Source: CAD feature listing. Evaluate the final solid. Frame: model axes, mm. Give positions to 0.01 mm unless a question says otherwise; leave off trailing zeros. Write each loop counter-clockwise with the first axis right and the second up, starting at its lowest first coordinate (ties: lowest second). Pieces come first, ordered by that corner, then holes. Notation, with made-up numbers: (4, 64.25) -> (33, 64.25) arc R5 ccw to (33, 72.25) -> close; hole circle Ø11 at (-15.75, 55.5). An arc over 180 degrees is marked (long way). Answer as a JSON object with one key per item and string values. Group by question number.
Item 1: Section query A-A on y = 0.75. Return the cut outline in (x, z), plus the area to 3 significant figures.
Item 2: Ray query, probe 1 along Z at (x, y) = (26, 2); probe 2 along Z at (x, y) = (-1, 2); probe 3 along X at (y, z) = (0.45, -1.5) (1 decimal). Return the intervals inside material, ascending. Write a range as from..to.
Item 3: First-contact query: pin 1 Ø2 at (x, y) = (23.5, 2) entering from +Z; pin 2 Ø2 at (x, y) = (6.5, 1) entering from +Z. Flat tips, straight axial feed; report the tip coordinate or a pass-through.
Item 4: Section query B-B on x = 4. Return the cut outline in (y, z).
Item 5: Section query C-C on z = -35. Return the cut outline in (x, y), plus the area to 3 significant figures.
Item 6: Section query D-D on x = 36. Return the cut outline in (y, z), plus the area to 3 significant figures.
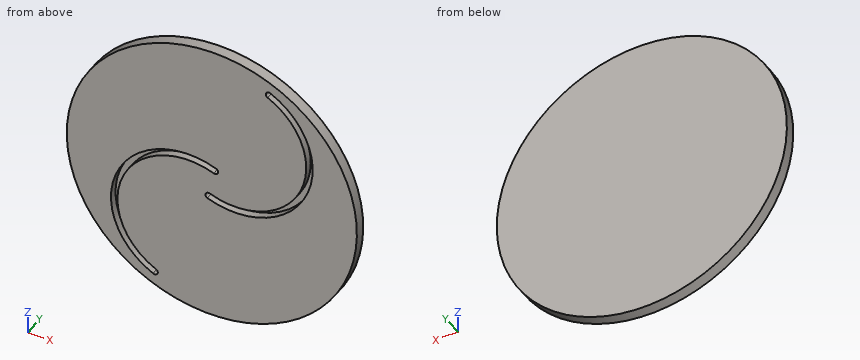
from build123d import *

# Parameters (mm, degrees)
SKETCH1_R           = 45
BOSS_EXTRUDE1_DEPTH = 3.5
CAVITY1_DEPTH       = 2.5


# Read off the part's stored shape, not the designer's step: Cavity1
with BuildPart() as part:
    # Sketch1 → Boss-Extrude1 (new body)
    with BuildSketch(Plane(origin=(0, 0, 0), x_dir=(1, 0, 0), z_dir=(0, 1, 0))):
        with Locations(Location((0, 0, 0), (0, 0, 270))):
            Circle(SKETCH1_R)
    extrude(amount=BOSS_EXTRUDE1_DEPTH)

    # Cavity1 outline → Cavity1 (cut)
    with BuildSketch(Plane(origin=(0, 0, 0), x_dir=(1, 0, 0), z_dir=(0, 1, 0))):
        with BuildLine():
            ThreePointArc((-1.897013309, 4.206804256), (-1.35975038, 3.69058849), (-0.614681205, 3.689140702))
            ThreePointArc((-0.614681205, 3.689140702), (27.363668078, -7.605415279), (17.306098008, -36.05186159))
            ThreePointArc((17.306098008, -36.05186159), (16.813923428, -36.611231194), (16.845129248, -37.355647991))
            ThreePointArc((16.845129248, -37.355647991), (17.423389863, -37.887377997), (18.207362086, -37.837281165))
            ThreePointArc((18.207362086, -37.837281165), (29.186869676, -6.783262051), (-1.356143814, 5.546621038))
            ThreePointArc((-1.356143814, 5.546621038), (-1.91270489, 4.992218741), (-1.897013309, 4.206804256))
        make_face()
        with BuildLine():
            ThreePointArc((1.897013309, -4.206804256), (1.35975038, -3.69058849), (0.614681205, -3.689140702))
            ThreePointArc((0.614681205, -3.689140702), (-27.363668078, 7.605415279), (-17.306098008, 36.05186159))
            ThreePointArc((-17.306098008, 36.05186159), (-16.813923428, 36.611231194), (-16.845129248, 37.355647991))
            ThreePointArc((-16.845129248, 37.355647991), (-17.423389863, 37.887377997), (-18.207362086, 37.837281165))
            ThreePointArc((-18.207362086, 37.837281165), (-29.186869676, 6.783262051), (1.356143814, -5.546621038))
            ThreePointArc((1.356143814, -5.546621038), (1.91270489, -4.992218741), (1.897013309, -4.206804256))
        make_face()
    extrude(amount=CAVITY1_DEPTH, mode=Mode.SUBTRACT)


solid = part.part
Worked answers:
{
 "1": {"outline": "circle Ø90 at (0, 0); hole (-18.21, -37.84) arc R1 ccw to (-17.31, -36.05) arc R21.82 cw to (0.61, 3.69) arc R1 ccw to (1.36, 5.55) arc R23.82 ccw to start; hole (-1.36, -5.55) arc R23.82 ccw to (18.21, 37.84) arc R1 ccw to (17.31, 36.05) arc R21.82 cw to (-0.61, -3.69) arc R1 ccw to start", "area": "6,080 mm^2"},
 "2": {"probe 1": "-36.73..1.6, 5.05..28.1, 31.54..36.73", "probe 2": "-44.99..-5.69, -3.62..4.26, 6.35..44.99", "probe 3": "-45..-25.9, -23.2..19.7, 23..45"},
 "3": {"pin 1": "z = 38.97", "pin 2": "z = 44.66"},
 "4": {"outline": "(0, -44.82) -> (3.5, -44.82) -> (3.5, 44.82) -> (0, 44.82) -> (0, -4.97) -> (2.5, -4.97) -> (2.5, -6.99) -> (0, -6.99) -> close"},
 "5": {"outline": "(-28.28, 0) -> (-22.57, 0) -> (-22.57, 2.5) -> (-19.16, 2.5) -> (-19.16, 0) -> (28.28, 0) -> (28.28, 3.5) -> (-28.28, 3.5) -> close", "area": "189 mm^2"},
 "6": {"outline": "(0, -27) -> (3.5, -27) -> (3.5, 27) -> (0, 27) -> close", "area": "189 mm^2"}
}
